Could you check a few things on this model? Use its own coordinates, in mm. Face numbers are marked on the shaded views. A direction names the side the tool comes from. Give positions to 0.01 mm unless a question says otherwise; leave off trailing zeros. Write each loop counter-clockwise with the first axis right and the second up, starting at its lowest first coordinate (ties: lowest second). Pieces come first, ordered by that corner, then holes. Notation, with made-up numbers: (-2, 46) - (11, 46) arc R14 cw to (11, 63) - close; hole circle Ø6 at (30.25, 24). An arc over 180 degrees is marked (long way). Answer in a Markdown table with one row per item.
from build123d import *

# Parameters (mm, degrees)
SKETCH1_R           = 9
BOSS_EXTRUDE3_DEPTH = 10
FILLET1_R           = 10
CUT_EXTRUDE2_DEPTH  = 10


with BuildPart() as part:
    # Sketch1 → Boss-Extrude3 (new body)
    with BuildSketch(Plane.XY):
        with BuildLine():
            Line((-58.704034486, 12.783450444), (67.393380319, 12.783450444))
            ThreePointArc((67.393380319, 12.783450444), (96.844672917, 0), (67.393380319, -12.783450444))
            Line((67.393380319, -12.783450444), (-58.704034486, -12.783450444))
            ThreePointArc((-58.704034486, -12.783450444), (-88.155327083, 0), (-58.704034486, 12.783450444))
        make_face()
        with Locations((-70.655327083, 0)):
            Circle(SKETCH1_R, mode=Mode.SUBTRACT)
        with Locations((79.344672917, 0)):
            Circle(SKETCH1_R, mode=Mode.SUBTRACT)
        with BuildLine():
            Line((-53.412978839, 6.702415671), (-39.501397037, 6.702415671))
            ThreePointArc((-39.501397037, 6.702415671), (-32.798981366, 0), (-39.501397037, -6.702415671))
            Line((-39.501397037, -6.702415671), (-53.412978839, -6.702415671))
            ThreePointArc((-53.412978839, -6.702415671), (-60.11539451, 0), (-53.412978839, 6.702415671))
        make_face(mode=Mode.SUBTRACT)
        with BuildLine():
            Line((-3.412978839, 6.702415671), (10.498602963, 6.702415671))
            ThreePointArc((10.498602963, 6.702415671), (17.201018634, 0), (10.498602963, -6.702415671))
            Line((10.498602963, -6.702415671), (-3.412978839, -6.702415671))
            ThreePointArc((-3.412978839, -6.702415671), (-10.11539451, 0), (-3.412978839, 6.702415671))
        make_face(mode=Mode.SUBTRACT)
        with BuildLine():
            Line((46.587021161, 6.702415671), (60.498602963, 6.702415671))
            ThreePointArc((60.498602963, 6.702415671), (67.201018634, 0), (60.498602963, -6.702415671))
            Line((60.498602963, -6.702415671), (46.587021161, -6.702415671))
            ThreePointArc((46.587021161, -6.702415671), (39.88460549, 0), (46.587021161, 6.702415671))
        make_face(mode=Mode.SUBTRACT)
    extrude(amount=BOSS_EXTRUDE3_DEPTH)

    # Fillet1
    fillet1_edges = [part.edges().sort_by_distance(p)[0] for p in [
        (67.393380319, -12.783450444, 5),
        (-58.704034486, -12.783450444, 5),
        (-58.704034486, 12.783450444, 5),
        (67.393380319, 12.783450444, 5),
    ]]
    fillet(fillet1_edges, radius=FILLET1_R)

    # Sketch4 → Cut-Extrude2 (cut)
    with BuildSketch(Plane.XY.offset(10)):
        Polygon((82.625844791, -8.343662686), (83.067179358, -9.178208957), (84.835179052, -8.243234581), (84.393844485, -7.40868831), align=None)
    extrude(amount=-CUT_EXTRUDE2_DEPTH, mode=Mode.SUBTRACT)


solid = part.part
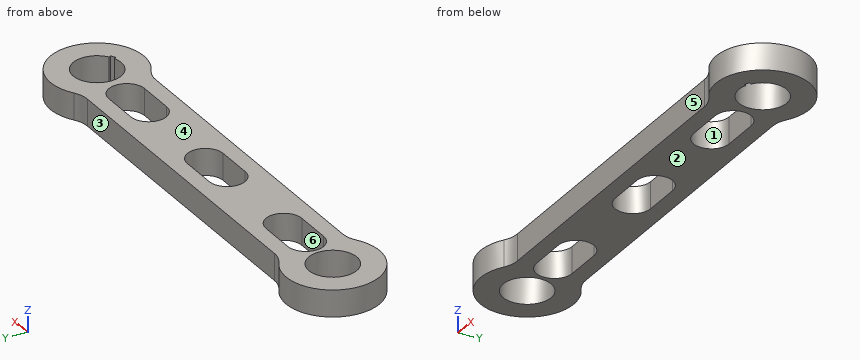
1) Imagine slicing it at D-D (y = 11). List the corners of the cut face in (x, z) for me.
Check values:
| item | result |
|---|---|
| outline | (-84.27, 0) - (92.96, 0) - (92.96, 10) - (-84.27, 10) - close |
2) Imagine slicing it at A-A (y = 0). List the corners of the cut face in (x, z) for me, then the cut area to 3 significant figures.
Check values:
| item | result |
|---|---|
| outline | (-88.16, 0) - (-79.66, 0) - (-79.66, 10) - (-88.16, 10) - close; (-61.66, 0) - (-60.12, 0) - (-60.12, 10) - (-61.66, 10) - close; (-32.8, 0) - (-10.12, 0) - (-10.12, 10) - (-32.8, 10) - close; (17.2, 0) - (39.88, 0) - (39.88, 10) - (17.2, 10) - close; (67.2, 0) - (70.34, 0) - (70.34, 10) - (67.2, 10) - close; (88.34, 0) - (96.84, 0) - (96.84, 10) - (88.34, 10) - close |
| area | 671 mm2 |
3) On a 3-axis mill with a long thin cutter (end or side, diameter ignored), from which of +Z, -Z, +X, -X, +Y, -Y can I reach the whole of each face in a straight line? I mean the marked faces 3, 4, 5 and 6. Say none if no direction works.
Check values:
| item | result |
|---|---|
| face 3 | +Z, -Z, +Y |
| face 4 | +Z, +X, -X, +Y, -Y |
| face 5 | +Z, -Z, -Y |
| face 6 | +Z, -Z |
4) We'd pull the mould along X, two halves only. Please class the marked faces 1 and 2: +X half, -X half, draft (parallel to the pull), parting line (faces both ways), or undercut.
Check values:
| item | result |
|---|---|
| face 1 | undercut |
| face 2 | draft |
5) If I drill on line 1 (Y direction, x = -3, z = 6.25); line 2 (X direction, y = 3.5, z = 8.25); line 3 (X direction, y = -2.5, z = 9.25), over which ranges is the centre line in solid material (lowest first)?
Check values:
| item | result |
|---|---|
| line 1 | y = -12.78 to -6.7, 6.7 to 12.78 |
| line 2 | x = -87.8 to -78.95, -62.36 to -59.13, -33.79 to -9.13, 16.21 to 40.87, 66.21 to 71.05, 87.64 to 96.49 |
| line 3 | x = -87.98 to -79.3, -62.01 to -59.63, -33.28 to -9.63, 16.72 to 40.37, 66.72 to 70.7, 87.99 to 96.67 |
6) Imagine slicing it at C-C (x = -1). List the corners of the cut face in (y, z) for me.
Check values:
| item | result |
|---|---|
| outline | (-12.78, 0) - (-6.7, 0) - (-6.7, 10) - (-12.78, 10) - close; (6.7, 0) - (12.78, 0) - (12.78, 10) - (6.7, 10) - close |
7) Imagine slicing it at B-B (z = 3.75). List the corners of the cut face in (x, y) for me, then the cut area to 3 significant figures.
Check values:
| item | result |
|---|---|
| outline | (-60.86, -14.5) arc R10 cw to (-55.26, -12.78) - (63.94, -12.78) arc R10 cw to (69.54, -14.5) arc R17.5 ccw (long way) to (69.54, 14.5) arc R10 cw to (63.94, 12.78) - (-55.26, 12.78) arc R10 cw to (-60.86, 14.5) arc R17.5 ccw (long way) to start; hole circle Ø18 at (-70.66, 0); hole (-53.41, -6.7) - (-39.5, -6.7) arc R6.7 ccw to (-39.5, 6.7) - (-53.41, 6.7) arc R6.7 ccw to start; hole (-3.41, -6.7) - (10.5, -6.7) arc R6.7 ccw to (10.5, 6.7) - (-3.41, 6.7) arc R6.7 ccw to start; hole (46.59, -6.7) - (60.5, -6.7) arc R6.7 ccw to (60.5, 6.7) - (46.59, 6.7) arc R6.7 ccw to start; hole (82.64, -8.37) - (83.07, -9.18) - (84.84, -8.24) - (84.41, -7.44) arc R9 ccw (long way) to start |
| area | 3,460 mm2 |
8) Will these pins go through, and if not, where does the flat tip stop? P1, Ø3, axis at x = 7.5, y = -12, coming from the -Z side; P2, Ø3, axis at x = 3.5, z = 3.5, coming from the +Y side; P3, Ø1.5, axis at y = -3.5, z = 8, coming from the -X side; P4, Ø3, axis at x = -0.5, z = 3.5, coming from the -Y side.
Check values:
| item | result |
|---|---|
| P1 | stops at z = 0 |
| P2 | stops at y = 12.78 |
| P3 | stops at x = -87.94 |
| P4 | stops at y = -12.78 |
